```python
from build123d import *

# Parameters (mm, degrees)
F2_DEPTH = 12.7
F1_W     = 38.9029346406
F1_H     = 32.7060050331
F3_DEPTH = 6.35
F4_R     = 5.08
F5_R     = 1.27


# Not quite as in the source:
# - two fillets or chamfers of one size are made in one step
# - a feature names something its author has since deleted; it is built from what else it names


with BuildPart() as f2:
    # F0 (on Front) → F2 (new body, symmetric)
    with BuildSketch(Plane.XZ):
        with BuildLine():
            Line((-80.5600658059, -3.4427349456), (0, -3.4427349456))
            Line((0, -3.4427349456), (0, 49.5754186995))
            Line((0, 49.5754186995), (-80.5600658059, 49.5754186995))
            ThreePointArc((-80.5600658059, 49.5754186995), (-92.446291157, 23.066341877), (-80.5600658059, -3.4427349456))
        make_face()
    extrude(amount=F2_DEPTH, both=True)

    # F1 (on Front) → F3 (join, symmetric)
    with BuildSketch(Plane.XZ):
        with Locations((19.4514673203, 23.5827539582)):
            Rectangle(F1_W, F1_H)
    extrude(amount=F3_DEPTH, both=True)

    # F4
    f4_edges = [f2.edges().sort_by_distance(p)[0] for p in [
        (-40.280033, -12.7, -3.442735),
        (-40.280033, -12.7, 49.575419),
        (-40.280033, 12.7, -3.442735),
        (-40.280033, 12.7, 49.575419),
        (-92.446291, 12.7, 23.066342),
        (-80.560066, 0, -3.442735),
        (-92.446291, -12.7, 23.066342),
        (-80.560066, 0, 49.575419),
        (0, 0, -3.442735),
        (0, 0, 49.575419),
    ]]
    fillet(f4_edges, radius=F4_R)

    # F5
    f5_edges = [f2.edges().sort_by_distance(p)[0] for p in [
        (19.451467, -6.35, 39.935756),
        (19.451467, -6.35, 7.229751),
        (19.451467, 6.35, 39.935756),
        (19.451467, 6.35, 7.229751),
    ]]
    fillet(f5_edges, radius=F5_R)


solid = f2.part
```
Can you work these out from the model? Positions are in its coordinate system, mm. A direction names the side the tool comes from. Give positions to 0.01 mm unless a question says otherwise; leave off trailing zeros. Write each loop counter-clockwise with the first axis right and the second up, starting at its lowest first coordinate (ties: lowest second). Pieces come first, ordered by that corner, then holes. Notation, with made-up numbers: (8.5, 37) - (12.5, 37) arc R16 cw to (12.5, 59) - close; hole circle Ø5 at (88.25, 14.25). An arc over 180 degrees is marked (long way). Write item = value, one per line. Start each with the question number.
1. Please list where these lines run through material, in increasing order: line 1 (Z direction, x = 21, y = 3); line 2 (Y direction, x = 9.5, z = 18); line 3 (Y direction, x = -1.5, z = 45).
2. For pin 1 (8 mm diameter, centred on x = 28.5, y = 1.5, fed in from -Z); pin 2 (2 mm diameter, centred on y = -2.5, z = 11.5, fed in from -X); pin 3 (3 mm diameter, centred on x = 12, y = 0.5, fed in from +Z), each with a flat end and sliding along its axis, tell me the tip position at first contact or that it passes through.
3. On a 3-axis mill with a long thin cutter (end or side, diameter ignored), from which of +Z, -Z, +X, -X, +Y, -Y can I reach the whole of each face in a straight line? I mean faces 1 (the face through (19, -6.35, 24)), 2 (the face through (19, 0, 7.23)), 3 (the face through (19, 0, 39.936)), 4 (the face through (-44, 12.7, 23)). Say none if no direction works.
4. Imagine slicing it at A-A (x = -38.5). Please give me the cut outline in (y, z), and give its area (3 significant figures).
5. Imagine slicing it at B-B (y = -2). Please give me the cut outline in (x, z).
6. Imagine slicing it at C-C (x = 20.5). Please give me the cut outline in (y, z).
Worked answers:
q1.line_1 = 7.23 to 39.94
q1.line_2 = -6.35 to 6.35
q1.line_3 = -12.67 to 12.67
q2.pin_1 = 7.23
q2.pin_2 = -90.84
q2.pin_3 = 39.94
q3.face_1 = +Z, -Z, +X, -Y
q3.face_2 = -Z, +X, +Y, -Y
q3.face_3 = +Z, +X, +Y, -Y
q3.face_4 = +Z, -Z, +X, -X, +Y
q4.outline = (-12.7, 1.64) arc R5.08 ccw to (-7.62, -3.44) - (7.62, -3.44) arc R5.08 ccw to (12.7, 1.64) - (12.7, 44.5) arc R5.08 ccw to (7.62, 49.58) - (-7.62, 49.58) arc R5.08 ccw to (-12.7, 44.5) - close
q4.area = 1,320 mm2
q5.outline = (-82.14, -1.94) arc R5.08 ccw to (-78.54, -3.44) - (-5.08, -3.44) arc R5.08 ccw to (0, 1.64) - (0, 7.23) - (38.9, 7.23) - (38.9, 39.94) - (0, 39.94) - (0, 44.5) arc R5.08 ccw to (-5.08, 49.58) - (-78.54, 49.58) arc R5.08 ccw to (-82.14, 48.07) arc R35.5 ccw to start
q6.outline = (-6.35, 8.5) arc R1.27 ccw to (-5.08, 7.23) - (5.08, 7.23) arc R1.27 ccw to (6.35, 8.5) - (6.35, 38.67) arc R1.27 ccw to (5.08, 39.94) - (-5.08, 39.94) arc R1.27 ccw to (-6.35, 38.67) - close
